```python
from build123d import *

# Parameters (mm, degrees)
BOSS_EXTRUDE1_DEPTH     = 22.225
FILLET1_R               = 25.4
CUT_EXTRUDE1_DEPTH      = 129.456170755
CUT_EXTRUDE1_DEPTH_BACK = 129.456170755
SKETCH2_W               = 58.42
SKETCH2_H               = 2.835975014
BOSS_EXTRUDE2_DEPTH     = 22.352
FILLET2_SIZE            = 3.175
FILLET2_SIZE_2          = 6.35
SKETCH4_R               = 5.715
SKETCH4_R_2             = 3.81
CUT_EXTRUDE2_DEPTH      = 3.175
FILLET4_R               = 1.27
SKETCH5_R               = 2.5
CUT_EXTRUDE3_DEPTH      = 110.417000644
CUT_EXTRUDE5_DEPTH      = 7
SKETCH8_R               = 2
BOSS_EXTRUDE3_DEPTH     = 6.35
FILLET3_R               = 3.175
SKETCH6_R               = 4.25
CUT_EXTRUDE8_DEPTH      = 24.13


with BuildPart() as part:
    # Sketch1 → Boss-Extrude1 (new, symmetric)
    with BuildSketch(Plane.XY):
        Polygon((-17.78, 72.220471881), (-17.78, 49.868471881), (-50.8, 49.868471881), (-50.8, 41.401805214), (-101.6, 41.401805214), (-20.955, 75.395471881), (50.8, 75.395471881), (50.8, 72.220471881), align=None)
    extrude(amount=BOSS_EXTRUDE1_DEPTH, both=True)

    # Fillet1
    fillet1_edges = [part.edges().sort_by_distance(p)[0] for p in [
        (-20.955, 75.395471881, 0),
    ]]
    fillet(fillet1_edges, radius=FILLET1_R)

    # Sketch3 → Cut-Extrude1 (cut, two sides: drawn at the far end of the back side and taken through both)
    with BuildSketch(Plane(origin=(-50.8, 0, 0), x_dir=(0, 0, -1), z_dir=(1, 0, 0)).offset(-CUT_EXTRUDE1_DEPTH_BACK)):
        with BuildLine():
            Line((-132.858425435, -9.823961327), (-22.225, 41.401805214))
            ThreePointArc((-22.225, 41.401805214), (0, 46.297479222), (22.225, 41.401805214))
            Line((22.225, 41.401805214), (132.858425435, -9.823961327))
            Line((132.858425435, -9.823961327), (132.858425435, -253.658610064))
            Line((132.858425435, -253.658610064), (-132.858425435, -253.658610064))
            Line((-132.858425435, -253.658610064), (-132.858425435, -9.823961327))
        make_face()
    extrude(amount=CUT_EXTRUDE1_DEPTH + CUT_EXTRUDE1_DEPTH_BACK, mode=Mode.SUBTRACT)

    # Sketch2 → Boss-Extrude2 (add)
    with BuildSketch(Plane.XZ.offset(-72.220471881)):
        with Locations((11.43, 20.807012493)):
            Rectangle(SKETCH2_W, SKETCH2_H)
        with Locations((11.43, -20.807012493)):
            Rectangle(SKETCH2_W, SKETCH2_H)
    extrude(amount=BOSS_EXTRUDE2_DEPTH)

    # Fillet2
    # an asymmetric fillet: 6.35, 3.175 mm, written as the material it takes off along each edge
    with BuildSketch(Plane(origin=(50.8, 75.395471881, -38.1), x_dir=(0, -1, 0), z_dir=(0, 0, 1))) as fillet2_piece_1:
        with BuildLine():
            Bezier((FILLET2_SIZE, 0), (0, 0), (0, -FILLET2_SIZE_2), weights=[1, 0.707106781, 1])
            Line((0, -FILLET2_SIZE_2), (0, 0))
            Line((0, 0), (FILLET2_SIZE, 0))
        make_face()
    extrude(amount=76.2, mode=Mode.SUBTRACT)

    # Sketch4 → Cut-Extrude2 (cut)
    with BuildSketch(Plane(origin=(0, 75.395471881, 0), x_dir=(1, 0, 0), z_dir=(0, 1, 0))):
        with Locations(Location((-7.110857048, 0, 0), (0, 0, 270))):
            Circle(SKETCH4_R)
        with Locations(Location((3.189142952, 0, 0), (0, 0, 270))):
            Circle(SKETCH4_R_2)
        with BuildLine():
            Line((9.34361728, 0.635), (12.39161728, 0.635))
            ThreePointArc((12.39161728, 0.635), (13.02661728, 0), (12.39161728, -0.635))
            Line((12.39161728, -0.635), (9.34361728, -0.635))
            ThreePointArc((9.34361728, -0.635), (8.70861728, 0), (9.34361728, 0.635))
        make_face()
    extrude(amount=-CUT_EXTRUDE2_DEPTH, mode=Mode.SUBTRACT)

    # Fillet4
    # the kernel refuses this fillet: 1.27 mm, written as the material it takes off along each edge
    with BuildSketch(Plane(origin=(-7.110857048, 75.395471881, 0), x_dir=(0, 0, 1), z_dir=(-1, 0, 0))) as fillet4_piece_1:
        with BuildLine():
            CenterArc((5.715 + FILLET4_R, -FILLET4_R), FILLET4_R, 90, 90)
            Line((5.715, -FILLET4_R), (5.715, 0))
            Line((5.715, 0), (5.715 + FILLET4_R, 0))
        make_face()
    revolve(axis=Axis((-7.110857048, 75.395471881, 0), (0, 1, 0)), mode=Mode.SUBTRACT)
    with BuildSketch(Plane(origin=(3.189142952, 75.395471881, 0), x_dir=(0, 0, 1), z_dir=(-1, 0, 0))) as fillet4_piece_2:
        with BuildLine():
            CenterArc((3.81 + FILLET4_R, -FILLET4_R), FILLET4_R, 90, 90)
            Line((3.81, -FILLET4_R), (3.81, 0))
            Line((3.81, 0), (3.81 + FILLET4_R, 0))
        make_face()
    revolve(axis=Axis((3.189142952, 75.395471881, 0), (0, 1, 0)), mode=Mode.SUBTRACT)

    # Sketch5 → Cut-Extrude3 (cut, through all)
    with BuildSketch(Plane(origin=(0, 75.395471881, 0), x_dir=(1, 0, 0), z_dir=(0, 1, 0))):
        with Locations(Location((-66.620425581, 0, 0), (0, 0, 270))):
            Circle(SKETCH5_R)
    extrude(amount=-CUT_EXTRUDE3_DEPTH, mode=Mode.SUBTRACT)

    # Sketch7 → Cut-Extrude5 (cut)
    with BuildSketch(Plane.XZ.offset(-49.868471881)):
        with BuildLine():
            Line((-38.862, 5), (-26.162, 5))
            ThreePointArc((-26.162, 5), (-21.162, 0), (-26.162, -5))
            Line((-26.162, -5), (-38.862, -5))
            ThreePointArc((-38.862, -5), (-43.862, 0), (-38.862, 5))
        make_face()
    extrude(amount=-CUT_EXTRUDE5_DEPTH, mode=Mode.SUBTRACT)

    # Sketch8 → Boss-Extrude3 (add)
    # profile 1 of 2: a face of its own
    with BuildSketch(Plane(origin=(40.64, 0, 0), x_dir=(0, 0, -1), z_dir=(1, 0, 0))):
        with BuildLine():
            Line((-22.225, 49.868471881), (-24.765, 49.868471881))
            ThreePointArc((-24.765, 49.868471881), (-28.265, 53.368471881), (-24.765, 56.868471881))
            Line((-24.765, 56.868471881), (-22.225, 56.868471881))
            Line((-22.225, 56.868471881), (-22.225, 49.868471881))
        make_face()
        with Locations(Location((-24.765, 53.368471881, 0), (0, 0, 90))):
            Circle(SKETCH8_R, mode=Mode.SUBTRACT)
    # profile 2 of 2: a face of its own
    with BuildSketch(Plane(origin=(40.64, 0, 0), x_dir=(0, 0, -1), z_dir=(1, 0, 0))):
        with BuildLine():
            Line((22.225, 56.868471881), (22.225, 49.868471881))
            Line((22.225, 49.868471881), (24.765, 49.868471881))
            ThreePointArc((24.765, 49.868471881), (28.265, 53.368471881), (24.765, 56.868471881))
            Line((24.765, 56.868471881), (22.225, 56.868471881))
        make_face()
        with Locations(Location((24.765, 53.368471881, 0), (0, 0, 270))):
            Circle(SKETCH8_R, mode=Mode.SUBTRACT)
    extrude(amount=-BOSS_EXTRUDE3_DEPTH)

    # Fillet3
    # the kernel refuses this fillet: 3.175 mm, written as the material it takes off along each edge
    with BuildSketch(Plane(origin=(-15.820425581, 75.395471881, -22.225), x_dir=(0, -1, 0), z_dir=(1, 0, 0))) as fillet3_piece_1:
        with BuildLine():
            CenterArc((FILLET3_R, -FILLET3_R), FILLET3_R, 90, 90)
            Line((0, -FILLET3_R), (0, 0))
            Line((0, 0), (FILLET3_R, 0))
        make_face()
    extrude(amount=68.207925581, mode=Mode.SUBTRACT)
    with BuildSketch(Plane(origin=(-15.820425581, 49.995471881, -22.225), x_dir=(0, 1, 0), z_dir=(1, 0, 0))) as fillet3_piece_2:
        with BuildLine():
            CenterArc((25.4 - FILLET3_R, FILLET3_R), FILLET3_R, 270, 90)
            Line((25.4 - FILLET3_R, 0), (25.4, 0))
            Line((25.4, 0), (25.4, FILLET3_R))
        make_face()
    revolve(axis=Axis((-15.820425581, 49.995471881, -22.225), (0, 0, 1)), revolution_arc=22.856508496, mode=Mode.SUBTRACT)
    with BuildSketch(Plane(origin=(-108.914251568, 38.318685, -22.225), x_dir=(0.38842459395806633, -0.921480512440991, 0), z_dir=(0.921480512440991, 0.38842459395806633, 0))) as fillet3_piece_3:
        with BuildLine():
            CenterArc((FILLET3_R, -FILLET3_R), FILLET3_R, 90, 90)
            Line((0, -FILLET3_R), (0, 0))
            Line((0, 0), (FILLET3_R, 0))
        make_face()
    extrude(amount=90.319697679, mode=Mode.SUBTRACT)
    with BuildSketch(Plane(origin=(-108.914251568, 38.318685, 22.225), x_dir=(0.38842459395806633, -0.921480512440991, 0), z_dir=(0.921480512440991, 0.38842459395806633, 0))) as fillet3_piece_4:
        with BuildLine():
            CenterArc((FILLET3_R, FILLET3_R), FILLET3_R, 180, 90)
            Line((0, FILLET3_R), (0, 0))
            Line((0, 0), (FILLET3_R, 0))
        make_face()
    extrude(amount=90.319697679, mode=Mode.SUBTRACT)
    with BuildSketch(Plane(origin=(-15.820425581, 49.995471881, 22.225), x_dir=(0, 1, 0), z_dir=(1, 0, 0))) as fillet3_piece_5:
        with BuildLine():
            CenterArc((25.4 - FILLET3_R, -FILLET3_R), FILLET3_R, 0, 90)
            Line((25.4, -FILLET3_R), (25.4, 0))
            Line((25.4, 0), (25.4 - FILLET3_R, 0))
        make_face()
    revolve(axis=Axis((-15.820425581, 49.995471881, 22.225), (0, 0, 1)), revolution_arc=22.856508496, mode=Mode.SUBTRACT)
    with BuildSketch(Plane(origin=(-15.820425581, 75.395471881, 22.225), x_dir=(0, -1, 0), z_dir=(1, 0, 0))) as fillet3_piece_6:
        with BuildLine():
            CenterArc((FILLET3_R, FILLET3_R), FILLET3_R, 180, 90)
            Line((0, FILLET3_R), (0, 0))
            Line((0, 0), (FILLET3_R, 0))
        make_face()
    extrude(amount=68.207925581, mode=Mode.SUBTRACT)

    # Sketch6 → Cut-Extrude8 (cut)
    with BuildSketch(Plane(origin=(0, 75.395471881, 0), x_dir=(1, 0, 0), z_dir=(0, 1, 0))):
        with Locations(Location((-66.620425581, 0, 0), (0, 0, 270))):
            Circle(SKETCH6_R)
    extrude(amount=-CUT_EXTRUDE8_DEPTH, mode=Mode.SUBTRACT)


solid = part.part
```
Geometry check sheet. Reference: the model listing, model coordinates, mm. A direction names the side the tool comes from. Coordinates: 2 decimals unless noted, no trailing zeros. Order: outer loops, then holes, each group sorted by start corner. A loop starts at its lowest first (then second) coordinate and runs counter-clockwise, first axis right, second up. Notation, with made-up numbers: (63, 38) - (77, 38) arc R15 ccw to (77, 52) - close; hole circle Ø3 at (-18, -15). An arc over 180 degrees is marked (long way). Answer as a JSON object with one key per item and string values. Group by question number.
Item 1: Depth check by flat-ended pin: pin 1 Ø2 at (x, z) = (39, 23.5) entering from +Y; pin 2 Ø13 at (x, z) = (-7.11, 0) entering from +Y; pin 3 Ø8 at (y, z) = (60.5, -21.5) entering from +X; pin 4 Ø6 at (x, z) = (3.19, 0) entering from -Y. Enter the tip coordinate at first touch or a pass-through.
Item 2: Draft check along X on faces 1 (the face through (-64.142, 48.786, -0.325)), 2 (the face through (17.02, 74.49, 21.27)), 3 (the face through (-62.52, 56.89, 21.27)). Enter one of: +X half, -X half, draft (parallel to the pull), parting line (faces both ways), or undercut.
Item 3: Scan lines: probe 1 along Z at (x, y) = (26, 63) (3 decimals); probe 2 along X at (y, z) = (52.75, 0); probe 3 along Y at (x, z) = (28.5, -9). Record each from-to range of solid material in increasing order.
Item 4: Tool access check on faces 4 (the face through (38, 56.868, 24)), 5 (the face through (11, 61, -19.389)), 6 (the face through (11, 74, -0.635)). Record the directions out of +Z, -Z, +X, -X, +Y, -Y that give a thin tool (end or side, any length) a straight path to the whole face; none if there is none.
Item 5: Sectioned sample at A-A, the plane x = 28.5. Record the cut outline in (y, z) (3 decimals).
Resolved:
{
 "1": {"pin 1": "y = 56.87", "pin 2": "y = 75.3", "pin 3": "x = 40.64", "pin 4": "through"},
 "2": {"face 1": "undercut", "face 2": "draft", "face 3": "-X half"},
 "3": {"probe 1": "-22.225 to -19.389, 19.389 to 22.225", "probe 2": "-74.68 to -70.87, -62.37 to -43.86, -21.16 to -17.78", "probe 3": "72.22 to 75.4"},
 "4": {"face 4": "+Z, +X, -X, +Y", "face 5": "+X, -Y", "face 6": "+Y, -Y"},
 "5": {"outline": "(49.868, -22.225) - (72.22, -22.225) arc R3.175 ccw to (75.395, -19.05) - (75.395, 19.05) arc R3.175 ccw to (72.22, 22.225) - (49.868, 22.225) - (49.868, 19.389) - (72.22, 19.389) - (72.22, -19.389) - (49.868, -19.389) - close"}
}
